Geometry check sheet. Reference: the model listing, model coordinates, mm. Face numbers are marked on the shaded views. A direction names the side the tool comes from. Round coordinates to 2 decimals unless told otherwise and drop trailing zeros. Order: outer loops, then holes, each group sorted by start corner. A loop starts at its lowest first (then second) coordinate and runs counter-clockwise, first axis right, second up. Notation, with made-up numbers: M -23,-17.5 L -9,-17.5 A19 cw -9,8.5 Z; hole C 63,0 d10. An arc over 180 degrees is marked long. Answer as a JSON object with one key per item and string values. Group by question number.
```python
from build123d import *

# Parameters (mm, degrees)
SKETCH1_R               = 16
BOSS_EXTRUDE1_DEPTH     = 30
SKETCH2_R               = 3.175
BOSS_EXTRUDE2_DEPTH     = 20.582030842
SKETCH3_W               = 10.714658548
SKETCH3_H               = 10.331992171
BOSS_EXTRUDE3_DEPTH     = 6.612030842
SKETCH5_R               = 2.469573247
BOSS_EXTRUDE4_DEPTH     = 28
SKETCH6_R               = 16
BOSS_EXTRUDE5_DEPTH     = 10
SKETCH6_2_R             = 16
SKETCH6_2_R_2           = 2.5
CUT_EXTRUDE_THIN1_DEPTH = 6


with BuildPart() as part:
    # Sketch1 → Boss-Extrude1 (new body)
    with BuildSketch(Plane.XY):
        Circle(SKETCH1_R)
    extrude(amount=BOSS_EXTRUDE1_DEPTH)

    # Sketch2 → Boss-Extrude2 (add)
    with BuildSketch(Plane(origin=(0, 0, 0), x_dir=(0, 0, -1), z_dir=(1, 0, 0))):
        with Locations((-14.73814173, 0.386884617)):
            Circle(SKETCH2_R)
    extrude(amount=BOSS_EXTRUDE2_DEPTH)

    # Sketch3 → Boss-Extrude3 (add)
    with BuildSketch(Plane(origin=(20.582030842, 0, 0), x_dir=(0, 0, -1), z_dir=(1, 0, 0))):
        with Locations((-14.79803719, 0.233851674)):
            Rectangle(SKETCH3_W, SKETCH3_H)
    extrude(amount=BOSS_EXTRUDE3_DEPTH)

    # Sketch4 one side → Revolve1 (revolve)
    with BuildSketch(Plane(origin=(0, 0, 0), x_dir=(-1, 0, 0), z_dir=(0, 0, -1))):
        with BuildLine():
            ThreePointArc((9.999952802, -0.030723799), (9.999988201, -0.015361918), (10, 0))
            ThreePointArc((10, 0), (-0.066566913, 9.99977844), (-9.999113769, -0.133130877))
            Line((-9.999113769, -0.133130877), (9.999952802, -0.030723799))
        make_face()
    revolve(axis=Axis((15.849507962, -0.163088364, 0), (-0.99998689, 0.005120526, 0)))

    # Sketch5 → Boss-Extrude4 (add)
    with BuildSketch(Plane(origin=(0, 0, 0), x_dir=(-1, 0, 0), z_dir=(0, 0, -1))):
        Circle(SKETCH5_R)
    extrude(amount=BOSS_EXTRUDE4_DEPTH)

    # Sketch6 → Boss-Extrude5 (add)
    with BuildSketch(Plane(origin=(0, 0, -28), x_dir=(-1, 0, 0), z_dir=(0, 0, -1))):
        Circle(SKETCH6_R)
    extrude(amount=-BOSS_EXTRUDE5_DEPTH)

    # Sketch6_2 → Cut-Extrude-Thin1 (cut)
    with BuildSketch(Plane(origin=(0, 0, -28), x_dir=(-1, 0, 0), z_dir=(0, 0, -1))):
        Circle(SKETCH6_2_R)
        Circle(SKETCH6_2_R_2, mode=Mode.SUBTRACT)
    extrude(amount=-CUT_EXTRUDE_THIN1_DEPTH, mode=Mode.SUBTRACT)


solid = part.part
```
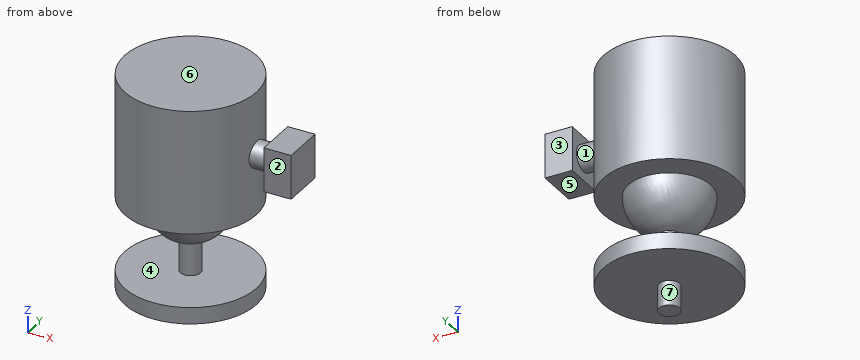
1) Sectioned sample at D-D (z = 8). Record the boundary of the cut face in (x, y), then the cut area to 3 significant figures.
2) Release check for a two-part mould opening along Z. For the marked faces 4, 5, 6 and 7 record: +Z half, -Z half, draft (parallel to the pull), parting line (faces both ways), or undercut.
3) Sectioned sample at A-A (y = 13.5). Record the boundary of the cut face in (x, z).
4) Set-up check for the marked faces 1, 2 and 3: record each of +Z, -Z, +X, -X, +Y, -Y from which the full face is reachable in a straight line by a thin tool's end or side.
5) Sectioned sample at C-C (z = 15). Record the boundary of the cut face in (x, y).
6) Sectioned sample at B-B (z = -10.5). Record the boundary of the cut face in (x, y), then the cut area to 3 significant figures.
7) Thickness scan on line 1 along Z through (x, y) = (4.5, 11); line 2 along X through (y, z) = (-0.5, 25); line 3 along X through (y, z) = (0.5, 15.5). Record the ranges inside material, lowest first. Write a range as [from, to].
8) Go/stop test with flat-tipped pins: P1, Ø7.5, axis at x = 24.5, z = 15, coming from the +Y side; P2, Ø7.5, axis at x = 23, y = -2.5, coming from the -Z side; P3, Ø3.5, axis at x = 24.5, y = 0, coming from the +Z side; P4, Ø1, axis at y = 11, z = -5.5, coming from the +X side. Record where each tip stops, or that it passes through.
Final values:
{
 "1": {"outline": "C 0,0 d32", "area": "804 mm^2"},
 "2": {"face 4": "undercut", "face 5": "-Z half", "face 6": "+Z half", "face 7": "draft"},
 "3": {"outline": "M -8.59,-22 L 8.59,-22 L 8.59,-18 L -8.59,-18 Z; M -8.59,0 L 8.59,0 L 8.59,30 L -8.59,30 Z"},
 "4": {"face 1": "none", "face 2": "+Z, -Z, +X, -Y", "face 3": "+Z, -Z, +X, +Y"},
 "5": {"outline": "M 15.6,3.55 A16 ccw long 15.76,-2.78 L 20.58,-2.78 L 20.58,-4.93 L 27.19,-4.93 L 27.19,5.4 L 20.58,5.4 L 20.58,3.55 Z"},
 "6": {"outline": "C 0,0 d4.94", "area": "19.2 mm^2"},
 "7": {"line 1": "z = [-22, -18], [0, 30]", "line 2": "x = [-15.99, 15.99]", "line 3": "x = [-15.99, 27.19]"},
 "8": {"P1": "stops at y = 5.4", "P2": "stops at z = 9.44", "P3": "stops at z = 20.16", "P4": "passes through"}
}
